Source: CAD feature listing. Evaluate the final solid. Frame: model axes, mm. Coordinates: 2 decimals unless noted, no trailing zeros. Loops run counter-clockwise (first coordinate to the right, second up) from the corner with the lowest first, then second, coordinate; pieces in that order, holes last.
Item 1: Section query A-A, the plane z = 3.2. Return the cut outline in (x, y), then the cut area to 3 significant figures.
Item 2: Section query B-B, the plane y = 4. Return the cut outline in (x, z), then the cut area to 3 significant figures.
Item 3: Line query: probe 1 along Y at (x, z) = (1.5, 4.05); probe 2 along X at (y, z) = (-1.25, 0.65); probe 3 along X at (y, z) = (0.5, 1.05). Output: solid intervals per line, ascending.
Item 4: Pin query (flat end, axial travel): pin 1 Ø1.5 at (y, z) = (0, 2.5) entering from +X; pin 2 Ø1 at (x, z) = (3.5, 4) entering from +Y. Return the tip coordinate at first contact, or that it passes through.
Item 5: Section query C-C, the plane x = 4.5. Return the cut outline in (y, z).
```python
from build123d import *

# Parameters (mm, degrees)
F3_DEPTH = 4.7625
F5_DEPTH = 4.7625


# Not quite as in the source:
# - the program builds the solid bodies; features that only make, move or delete a surface that nothing else refers to are left out


with BuildPart() as f3:
    # F0 (on Top) → F3 (new body)
    with BuildSketch(Plane.XY):
        Polygon((-2.7899552341, 4.7392185946), (-5.499261314, -0.0465628108), (-2.70930608, -4.7857814054), (2.7899552341, -4.7392185946), (5.499261314, 0.0465628108), (2.70930608, 4.7857814054), align=None)
    extrude(amount=F3_DEPTH)


with BuildPart() as f5:
    # F0 (on Top) → F5 (new body)
    with BuildSketch(Plane.XY):
        Polygon((-2.7899552341, 4.7392185946), (-5.499261314, -0.0465628108), (-2.70930608, -4.7857814054), (2.7899552341, -4.7392185946), (5.499261314, 0.0465628108), (2.70930608, 4.7857814054), align=None)
    extrude(amount=F5_DEPTH)


solid = f5.part
```
Verdict:
1. outline: (-5.5, -0.05) - (-2.71, -4.79) - (2.79, -4.74) - (5.5, 0.05) - (2.71, 4.79) - (-2.79, 4.74) - close
1. area: 78.6 mm2
2. outline: (-3.21, 0) - (3.17, 0) - (3.17, 4.76) - (-3.21, 4.76) - close
2. area: 30.4 mm2
3. probe 1: y = -4.75 to 4.78
3. probe 2: x = -4.79 to 4.77
3. probe 3: x = -5.19 to 5.23
4. pin 1: stops at x = 5.5
4. pin 2: stops at y = 4.29
5. outline: (-1.72, 0) - (1.74, 0) - (1.74, 4.76) - (-1.72, 4.76) - close
